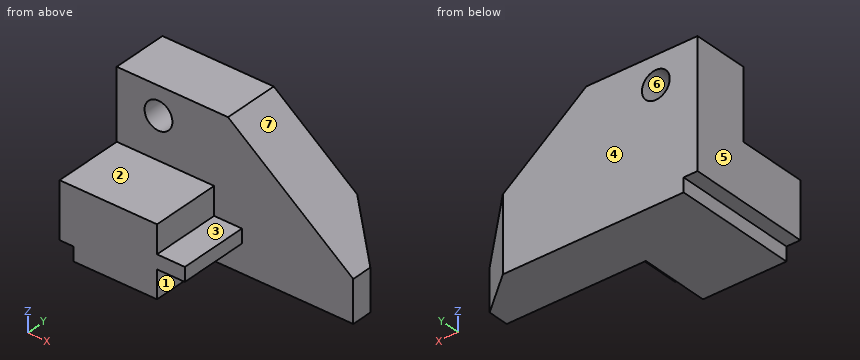
```python
from build123d import *

# Parameters (mm, degrees)
F1_DEPTH = 31.75
F2_R     = 6.35
F3_DEPTH = 25.4
F5_DEPTH = 63.501
F6_W     = 6.35
F6_H     = 6.35
F7_DEPTH = 57.151


with BuildPart() as f1:
    # F0 (on Front) → F1 (new body)
    with BuildSketch(Plane.XZ):
        Polygon((0, 31.75), (0, 0), (44.45, 0), (44.45, 12.7), (57.15, 12.7), (57.15, 19.05), (44.45, 19.05), (44.45, 31.75), align=None)
    extrude(amount=F1_DEPTH)

    # F2 (on Front) → F3 (join)
    with BuildSketch(Plane.XZ):
        Polygon((0, 63.5), (0, 0), (107.95, 0), (107.95, 19.05), (50.8, 63.5), align=None)
        with Locations((19.05, 50.8)):
            Circle(F2_R, mode=Mode.SUBTRACT)
    extrude(amount=-F3_DEPTH)

    # F4 (on Top) → F5 (cut, through all)
    with BuildSketch(Plane.XY):
        Polygon((107.95, 25.4), (88.9, 25.4), (107.95, 9.525), align=None)
    extrude(amount=F5_DEPTH, mode=Mode.SUBTRACT)

    # F6 (on face) → F7 (cut, through all)
    with BuildSketch(Plane.XZ.offset(31.75)):
        with Locations((3.175, 3.175)):
            Rectangle(F6_W, F6_H)
    extrude(amount=-F7_DEPTH, mode=Mode.SUBTRACT)


solid = f1.part
```
Geometry: final body of the model. Coordinates: model frame, mm. Face numbers are marked on the shaded views. A direction names the side the tool comes from. Give positions to 0.01 mm unless a question says otherwise; leave off trailing zeros. Loops run counter-clockwise (first coordinate to the right, second up) from the corner with the lowest first, then second, coordinate; pieces in that order, holes last. Notation, with made-up numbers: (-21, 85) -> (14, 85) arc R10 cw to (14, 101) -> close; hole circle Ø5 at (61, 51). An arc over 180 degrees is marked (long way). Use CSV: the item, a comma, the result in double quotes.
(1) Pull-direction query (Z, two-part tool) for the marked faces 5, 6 and 7; classes: released by +Z, released by -Z, zero draft, split by the parting line, or undercut.
From the geometry:
face 5,"zero draft"
face 6,"undercut"
face 7,"released by +Z"
(2) Cut plane D-D (x = 80). Output: boundary loops of the cut face in (y, z), plus the area to 3 significant figures.
From the geometry:
outline,"(0, 0) -> (25.4, 0) -> (25.4, 40.79) -> (0, 40.79) -> close"
area,"1,040 mm^2"
(3) First-contact query: P1, Ø2, axis at x = 60, y = 2, coming from the -Z side; P2, Ø14, axis at y = -14.5, z = 22.5, coming from the +X side; P3, Ø3, axis at y = 1.5, z = 39, coming from the +X side; P4, Ø14.5, axis at x = 19.05, z = 50.8, coming from the -Y side. Flat tips, straight axial feed; report the tip coordinate or a pass-through.
From the geometry:
P1,"z = 0"
P2,"x = 57.15"
P3,"x = 84.23"
P4,"y = 0"
(4) Access query for the marked faces 1, 2, 3 and 4. Directions: +Z, -Z, +X, -X, +Y, -Y. A direction counts if a zero-diameter tool reaches every point of the face in a straight line with its end or side. Return the directions, or none.
From the geometry:
face 1,"-Z, +X, -Y"
face 2,"+Z, +X, -X, -Y"
face 3,"+Z, +X, -Y"
face 4,"+Z, -Z, +X, -X, +Y"
(5) Ray query, line 1 along Z through (x, y) = (19, 10); line 2 along Y through (x, z) = (55, 8); line 3 along Z through (x, y) = (6.5, -2.5). Return the intervals inside material, ascending. Write a range as [from, to].
From the geometry:
line 1,"[0, 44.45], [57.15, 63.5]"
line 2,"[0, 25.4]"
line 3,"[0, 31.75]"
(6) Cut plane A-A (x = 19.05). Output: boundary loops of the cut face in (y, z).
From the geometry:
outline,"(-31.75, 0) -> (25.4, 0) -> (25.4, 44.45) -> (0, 44.45) -> (0, 31.75) -> (-31.75, 31.75) -> close; (0, 57.15) -> (25.4, 57.15) -> (25.4, 63.5) -> (0, 63.5) -> close"
(7) Cut plane C-C (z = 50.8). Output: boundary loops of the cut face in (x, y), plus the area to 3 significant figures.
From the geometry:
outline,"(0, 0) -> (12.7, 0) -> (12.7, 25.4) -> (0, 25.4) -> close; (25.4, 0) -> (67.13, 0) -> (67.13, 25.4) -> (25.4, 25.4) -> close"
area,"1,380 mm^2"
(8) Cut plane B-B (z = 10). Output: boundary loops of the cut face in (x, y) (3 decimals).
From the geometry:
outline,"(0, -31.75) -> (44.45, -31.75) -> (44.45, 0) -> (107.95, 0) -> (107.95, 9.525) -> (88.9, 25.4) -> (0, 25.4) -> close"
